```python
from build123d import *

# Parameters (mm, degrees)
BOSS_EXTRUDE1_DEPTH = 6
SKETCH3_W           = 48.26
SKETCH3_H           = 30.48
BOSS_EXTRUDE2_DEPTH = 6
CHAMFER1_SIZE       = 0.635
FILLET1_R           = 10
SKETCH4_W           = 31.3944
SKETCH4_H           = 6.3444
CUT_EXTRUDE1_DEPTH  = 73.882968029
FILLET2_R           = 1.27


with BuildPart() as part:
    # Sketch1 → Boss-Extrude1 (new body)
    with BuildSketch(Plane.XY):
        Polygon((28.6385, 47.625), (28.6385, 41.0972), (34.6329, 41.0972), (34.6329, 38.1), (37.8079, 38.1), (37.8079, 41.0972), (40.9829, 41.0972), (40.9829, 35.1028), (28.6385, 35.1028), (28.6385, 15.6972), (40.9829, 15.6972), (40.9829, 9.7028), (37.8079, 9.7028), (37.8079, 12.7), (34.6329, 12.7), (34.6329, 9.7028), (28.6385, 9.7028), (28.6385, 3.175), (15.8115, -47.625), (9.2837, -47.625), (9.2837, -53.6194), (6.2865, -53.6194), (6.2865, -56.7944), (9.2837, -56.7944), (9.2837, -59.9694), (3.2893, -59.9694), (3.2893, -47.625), (-16.1163, -47.625), (-16.1163, -59.9694), (-22.1107, -59.9694), (-22.1107, -56.7944), (-19.1135, -56.7944), (-19.1135, -53.6194), (-22.1107, -53.6194), (-22.1107, -47.625), (-28.6385, -47.625), align=None)
    extrude(amount=BOSS_EXTRUDE1_DEPTH)

    # Sketch3 → Boss-Extrude2 (add)
    with BuildSketch(Plane.XY.offset(6)):
        with Locations((0, -32.385)):
            Rectangle(SKETCH3_W, SKETCH3_H)
    extrude(amount=-BOSS_EXTRUDE2_DEPTH)

    # Chamfer1
    # the kernel refuses this chamfer: 0.635 mm, written as the material it adds along each edge
    with BuildSketch(Plane(origin=(23.5077, -17.145, 6), x_dir=(0.9995260143911436, -0.0307854926118649, 0), z_dir=(0, 0, -1))) as chamfer1_piece_1_section:
        Polygon((CHAMFER1_SIZE * 0.999526014391, -CHAMFER1_SIZE * 0.0307854926119), (CHAMFER1_SIZE * 0.214851580859, -CHAMFER1_SIZE * 0.976646711049), (0, 0), align=None)
    chamfer1_piece_1 = extrude(amount=6, mode=Mode.PRIVATE)
    chamfer1_piece_1 = split(chamfer1_piece_1, bisect_by=Plane(origin=(24.13, -16.940914613, 3), z_dir=(-1, 0, 0)), keep=Keep.TOP, mode=Mode.PRIVATE)
    add(chamfer1_piece_1)

    # Fillet1
    fillet1_edges = [part.edges().sort_by_distance(p)[0] for p in [
        (-10.30986, -17.145, 3),
        (-24.13, -40.127494457, 3),
    ]]
    fillet(fillet1_edges, radius=FILLET1_R)

    # Sketch4 → Cut-Extrude1 (cut, through all)
    with BuildSketch(Plane.XY.offset(6)):
        with Locations((-6.4135, -56.7972)):
            Rectangle(SKETCH4_W, SKETCH4_H)
    extrude(amount=-CUT_EXTRUDE1_DEPTH, mode=Mode.SUBTRACT)

    # Fillet2
    fillet2_edges = [part.edges().sort_by_distance(p)[0] for p in [
        (-16.1163, -53.625, 3),
        (3.2893, -53.625, 3),
        (9.2837, -53.6194, 3),
        (-22.1107, -53.6194, 3),
    ]]
    fillet(fillet2_edges, radius=FILLET2_R)


solid = part.part
```
Work out the finished part from the listing and answer in its coordinate system (mm). A direction names the side the tool comes from. Give positions to 0.01 mm unless a question says otherwise; leave off trailing zeros. Loops run counter-clockwise (first coordinate to the right, second up) from the corner with the lowest first, then second, coordinate; pieces in that order, holes last. Notation, with made-up numbers: (68, 14) -> (119, 14) arc R18 cw to (119, 26) -> close; hole circle Ø3 at (-21, 67.25). An arc over 180 degrees is marked (long way). Use CSV: the item, a comma, the result in double quotes.
1. Flat-ended cylindrical pins translate along their axes: pin 1 Ø1.8 at (y, z) = (-30.5, 3) entering from -X; pin 2 Ø3 at (x, z) = (-1, 3) entering from +Y; pin 3 Ø2 at (x, z) = (2.5, 2) entering from -Y; pin 4 Ø12 at (x, y) = (-7.5, -28.5) entering from -Z. Find the tip coordinate at first contact, or state that the pin passes through.
Found:
pin 1,"x = -24.13"
pin 2,"y = 0.83"
pin 3,"y = -53.06"
pin 4,"z = 0"
2. A tool of negligible diameter and unlimited length cuts with its end or side. For faces 5 (the flat face through (-22.111, -50, 3)), 6 (the flat face through (34.633, 11, 3)), 7 (the flat face through (17, -47.625, 3)), 8 (the flat face through (35, 15.697, 3)), from which of +Z, -Z, +X, -X, +Y, -Y can it reach the whole face along a straight path? Write none if from no direction.
Found:
face 5,"+Z, -Z, -X, -Y"
face 6,"+Z, -Z, -Y"
face 7,"+Z, -Z, +X, -Y"
face 8,"+Z, -Z, +X"
3. The part is cut by section B-B (x = -9.5). Write down the section's boundary in (y, z) (3 decimals), then the cut area to 3 significant figures.
Found:
outline,"(-47.625, 0) -> (-14.774, 0) -> (-14.774, 6) -> (-47.625, 6) -> close"
area,"197 mm^2"
4. The mould has two halves that part along X. Classify faces 1 (the flat face through (26.186, -6.539, 2.958)), 2 (the flat face through (-20, -17.145, 3)), 3 (the flat face through (34.633, 40, 3)), 4 (the flat face through (37.808, 40, 3)): +X half, -X half, draft (parallel to the pull), parting line (faces both ways), or undercut.
Found:
face 1,"+X half"
face 2,"draft"
face 3,"undercut"
face 4,"undercut"
5. The part is cut by section A-A (y = 30). Write down the section's boundary in (x, z).
Found:
outline,"(18.04, 0) -> (28.64, 0) -> (28.64, 6) -> (18.04, 6) -> close"
6. Straight lines are drawn through the part: line 1 (X direction, y = -32.5, z = 0.8); line 2 (Y direction, x = 38.5, z = 4.9); line 3 (Y direction, x = -24, z = 1.1) (3 decimals). For each, find the intervals that lie inside material, in ascending order.
Found:
line 1,"-24.13 to 24.13"
line 2,"9.7 to 15.7, 35.1 to 41.1"
line 3,"-47.625 to -17.145"
